Source: CAD feature listing. Evaluate the final solid. Frame: model axes, mm. A direction names the side the tool comes from. Give positions to 0.01 mm unless a question says otherwise; leave off trailing zeros. Write each loop counter-clockwise with the first axis right and the second up, starting at its lowest first coordinate (ties: lowest second). Pieces come first, ordered by that corner, then holes. Notation, with made-up numbers: M 64.25,80.25 L 84.25,80.25 A18 cw 84.25,111.25 Z; hole C 40.25,37 d8. An arc over 180 degrees is marked long. Return JSON: item names as keys, results as strings.
```python
from build123d import *

# Parameters (mm, degrees)
SKIZZE2_R                       = 3.25
SKIZZE2_R_2                     = 2.5
AUFSATZ_LINEAR_AUSTRAGEN1_DEPTH = 10
SKIZZE3_R                       = 1.25
AUFSATZ_LINEAR_AUSTRAGEN2_DEPTH = 2


with BuildPart() as part:
    # Skizze1 → Rotation1 (revolve)
    with BuildSketch(Plane.XY):
        Polygon((0, 0), (12.1, 0), (12.1, 30.8), (13.5, 30.8), (13.5, 60.8), (3.25, 60.8), (3.25, 70.8), (2.5, 70.8), (2.5, 62.8), (0, 62.8), align=None)
    revolve(axis=Axis((0, 12.380405046, 0), (0, -1, 0)))

    # Skizze2 → Aufsatz-Linear austragen1 (add)
    with BuildSketch(Plane(origin=(0, 60.8, 0), x_dir=(1, 0, 0), z_dir=(0, 1, 0))):
        with Locations((10, 0)):
            Circle(SKIZZE2_R)
        with Locations((10, 0)):
            Circle(SKIZZE2_R_2, mode=Mode.SUBTRACT)
    extrude(amount=AUFSATZ_LINEAR_AUSTRAGEN1_DEPTH)

    # Skizze3 → Aufsatz-Linear austragen2 (add)
    with BuildSketch(Plane(origin=(0, 60.8, 0), x_dir=(1, 0, 0), z_dir=(0, 1, 0))):
        with BuildLine():
            Line((-13.351029923, 2), (-18, 2))
            Line((-18, 2), (-18, -2))
            Line((-18, -2), (-13.351029923, -2))
            ThreePointArc((-13.351029923, -2), (-13.5, 0), (-13.351029923, 2))
        make_face()
        with Locations((-16, 0)):
            Circle(SKIZZE3_R, mode=Mode.SUBTRACT)
        with BuildLine():
            Line((18, -2), (13.351029923, -2))
            ThreePointArc((13.351029923, -2), (13.5, 0), (13.351029923, 2))
            Line((13.351029923, 2), (18, 2))
            Line((18, 2), (18, -2))
        make_face()
        with Locations((16, 0)):
            Circle(SKIZZE3_R, mode=Mode.SUBTRACT)
    extrude(amount=-AUFSATZ_LINEAR_AUSTRAGEN2_DEPTH)


solid = part.part
```
1) Draft query along Z for faces 1 (the face through (-0.54, 66.74, -2.44)), 2 (the face through (-16, 60, -2)), 3 (the face through (2.1, 30.8, 12.1)). Return one class per face: released by +Z, released by -Z, zero draft, split by the parting line, or undercut.
Numbers:
{"face 1": "undercut", "face 2": "released by -Z", "face 3": "zero draft"}
2) Cut plane C-C, the plane y = 38.5. Return the cut outline in (x, z).
Numbers:
{"outline": "C 0,0 d27"}
3) Set-up query: faces 4 (the face through (10, 60.8, 0)), 5 (the face through (-16, 60, 2)), 6 (the face through (16, 60, -2)), 7 (the face through (16, 60, 2)). Return all of +Z, -Z, +X, -X, +Y, -Y with unobstructed straight access to the full face (end or side cutting, diameter ignored); none if empty.
Numbers:
{"face 4": "+Y", "face 5": "+Z, -X, +Y, -Y", "face 6": "-Z, +X, +Y, -Y", "face 7": "+Z, +X, +Y, -Y"}
4) Cut plane B-B, the plane x = 0. Return the cut outline in (y, z).
Numbers:
{"outline": "M 0,-12.1 L 30.8,-12.1 L 30.8,-13.5 L 60.8,-13.5 L 60.8,-3.25 L 70.8,-3.25 L 70.8,-2.5 L 62.8,-2.5 L 62.8,2.5 L 70.8,2.5 L 70.8,3.25 L 60.8,3.25 L 60.8,13.5 L 30.8,13.5 L 30.8,12.1 L 0,12.1 Z"}
5) Contact query for flat-ended pins moving along their axis: pin 1 Ø8 at (y, z) = (16, -6) entering from -X; pin 2 Ø1.2 at (x, z) = (-16, 0.5) entering from -Y; pin 3 Ø12 at (x, z) = (2, 10) entering from -Y; pin 4 Ø5 at (y, z) = (20.5, -10.5) entering from -X. Output: stop coordinate, or through.
Numbers:
{"pin 1": "stops at x = -11.93", "pin 2": "passes through", "pin 3": "stops at y = 0", "pin 4": "stops at x = -9.08"}
6) Line query: line 1 (X direction, y = 60.15, z = 0); line 2 (Z direction, x = 10, y = 65.75); line 3 (Z direction, x = -16, y = 59). Output: solid intervals per line, ascending. Write a range as [from, to].
Numbers:
{"line 1": "x = [-18, -17.25], [-14.75, 14.75], [17.25, 18]", "line 2": "z = [-3.25, -2.5], [2.5, 3.25]", "line 3": "z = [-2, -1.25], [1.25, 2]"}
7) Cut plane D-D, the plane z = 4.25. Return the cut outline in (x, y), then the cut area to 3 significant figures.
Numbers:
{"outline": "M -12.81,30.8 L -11.33,30.8 L -11.33,0 L 11.33,0 L 11.33,30.8 L 12.81,30.8 L 12.81,60.8 L -12.81,60.8 Z", "area": "1,470 mm²"}
8) Cut plane A-A, the plane x = 16. Return the cut outline in (y, z), then the cut area to 3 significant figures.
Numbers:
{"outline": "M 58.8,-2 L 60.8,-2 L 60.8,-1.25 L 58.8,-1.25 Z; M 58.8,1.25 L 60.8,1.25 L 60.8,2 L 58.8,2 Z", "area": "3.00 mm²"}
